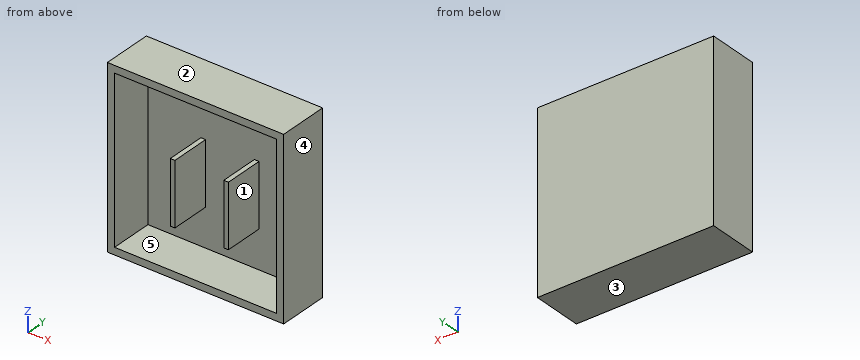
```python
from build123d import *

# Parameters (mm, degrees)
CROQUIS1_W              = 98.2
CROQUIS1_H              = 98.2
SALIENTE_EXTRUIR2_DEPTH = 28
CROQUIS2_W              = 90.2
CROQUIS2_H              = 90.2
CORTAR_EXTRUIR1_DEPTH   = 24
CROQUIS3_W              = 2.6
CROQUIS3_H              = 35
SALIENTE_EXTRUIR3_DEPTH = 22
CROQUIS5_W              = 2.6
CROQUIS5_H              = 35
SALIENTE_EXTRUIR4_DEPTH = 22


with BuildPart() as part:
    # Croquis1 → Saliente-Extruir2 (new body)
    with BuildSketch(Plane(origin=(0, 0, 0), x_dir=(1, 0, 0), z_dir=(0, 1, 0))):
        Rectangle(CROQUIS1_W, CROQUIS1_H)
    extrude(amount=-SALIENTE_EXTRUIR2_DEPTH)

    # Croquis2 → Cortar-Extruir1 (cut)
    with BuildSketch(Plane.XZ.offset(28)):
        Rectangle(CROQUIS2_W, CROQUIS2_H)
    extrude(amount=-CORTAR_EXTRUIR1_DEPTH, mode=Mode.SUBTRACT)

    # Croquis3 → Saliente-Extruir3 (add)
    with BuildSketch(Plane.XZ.offset(4)):
        with Locations((-14.3, -6.4)):
            Rectangle(CROQUIS3_W, CROQUIS3_H)
    extrude(amount=SALIENTE_EXTRUIR3_DEPTH)

    # Croquis5 → Saliente-Extruir4 (add)
    with BuildSketch(Plane.XZ.offset(4)):
        with Locations((15.49, -6.4)):
            Rectangle(CROQUIS5_W, CROQUIS5_H)
    extrude(amount=SALIENTE_EXTRUIR4_DEPTH)


solid = part.part
```
Geometry: final body of the model. Coordinates: model frame, mm. Face numbers are marked on the shaded views. A direction names the side the tool comes from. Coordinates: 2 decimals unless noted, no trailing zeros. Write each loop counter-clockwise with the first axis right and the second up, starting at its lowest first coordinate (ties: lowest second). Pieces come first, ordered by that corner, then holes. Notation, with made-up numbers: M -21,6 L 9,6 A21 ccw 9,26 Z; hole C -16,-7.5 d1. An arc over 180 degrees is marked long. Answer as CSV lines item,"result". Start each with the question number.
Q1. Line query: line 1 (Z direction, x = -14, y = -20.75); line 2 (X direction, y = -21, z = -13); line 3 (X direction, y = -19.25, z = 38). Output: solid intervals per line, ascending. Write a range as from..to.
Q2. Cut plane B-B on z = 39. Return the cut outline in (x, y), then the cut area to 3 significant figures.
Q3. Reachability of the marked faces 1 and 2 from +Z, -Z, +X, -X, +Y, -Y: full face, straight path, thin tool, end or side. Return the list, or none.
Q4. Cut plane D-D on z = -22.5. Return the cut outline in (x, y).
Q5. Mould query, pull axis Z, two halves, no side actions, for the marked faces 3, 4 and 5. Classes: released by +Z, released by -Z, zero draft, split by the parting line, or undercut.
Q6. Cut plane A-A on y = -8. Return the cut outline in (x, z), then the cut area to 3 significant figures.
Q7. Pin query (flat end, axial travel): P1, Ø4, axis at x = -3.5, z = 28, coming from the -Y side; P2, Ø3, axis at x = -14, z = -7.5, coming from the -Y side. Return the tip coordinate at first contact, or that it passes through.
Q8. Cut plane C-C on x = -33. Return the cut outline in (y, z).
Findings below:
1,line 1,"z = -49.1..-45.1, -23.9..11.1, 45.1..49.1"
1,line 2,"x = -49.1..-45.1, -15.6..-13, 14.19..16.79, 45.1..49.1"
1,line 3,"x = -49.1..-45.1, 45.1..49.1"
2,outline,"M -49.1,-28 L -45.1,-28 L -45.1,-4 L 45.1,-4 L 45.1,-28 L 49.1,-28 L 49.1,0 L -49.1,0 Z"
2,area,"585 mm2"
3,face 1,"-Y"
3,face 2,"+Z, +X, -X, +Y, -Y"
4,outline,"M -49.1,-28 L -45.1,-28 L -45.1,-4 L -15.6,-4 L -15.6,-26 L -13,-26 L -13,-4 L 14.19,-4 L 14.19,-26 L 16.79,-26 L 16.79,-4 L 45.1,-4 L 45.1,-28 L 49.1,-28 L 49.1,0 L -49.1,0 Z"
5,face 3,"released by -Z"
5,face 4,"zero draft"
5,face 5,"undercut"
6,outline,"M -49.1,-49.1 L 49.1,-49.1 L 49.1,49.1 L -49.1,49.1 Z; M -15.6,-23.9 L -13,-23.9 L -13,11.1 L -15.6,11.1 Z; M 14.19,-23.9 L 16.79,-23.9 L 16.79,11.1 L 14.19,11.1 Z; hole M -45.1,-45.1 L 45.1,-45.1 L 45.1,45.1 L -45.1,45.1 Z"
6,area,"1,690 mm2"
7,P1,"stops at y = -4"
7,P2,"stops at y = -26"
8,outline,"M -28,-49.1 L 0,-49.1 L 0,49.1 L -28,49.1 L -28,45.1 L -4,45.1 L -4,-45.1 L -28,-45.1 Z"
